Source: CAD feature listing. Evaluate the final solid. Frame: model axes, mm. A direction names the side the tool comes from. Give positions to 0.01 mm unless a question says otherwise; leave off trailing zeros. Loops run counter-clockwise (first coordinate to the right, second up) from the corner with the lowest first, then second, coordinate; pieces in that order, holes last. Notation, with made-up numbers: (-23.75, -25.75) -> (-6.75, -25.75) arc R8 cw to (-6.75, -15.75) -> close; hole circle Ø10 at (-24.5, 63.25). An arc over 180 degrees is marked (long way). Put each result on its own line as item: value.
```python
from build123d import *

# Parameters (mm, degrees)
SKETCH_1_W          = 48
SKETCH_1_H          = 69
EXTRUDE_1_DEPTH     = 2
SKETCH_2_W          = 60
SKETCH_2_H          = 81
EXTRUDE_2_DEPTH     = 2
SKETCH_3_W          = 48
SKETCH_3_H          = 69
CUT_EXTRUDE_1_DEPTH = 2
SKETCH_4_W          = 6
SKETCH_4_H          = 6
EXTRUDE_3_DEPTH     = 2
SKETCH_5_R          = 1.275
CUT_EXTRUDE_2_DEPTH = 2
FILLET_1_R          = 2


with BuildPart() as part:
    # 草图1 → 凸台-拉伸1 (new body)
    with BuildSketch(Plane(origin=(0, 0, 0), x_dir=(1, 0, 0), z_dir=(0, 1, 0))):
        Rectangle(SKETCH_1_W, SKETCH_1_H)
    extrude(amount=EXTRUDE_1_DEPTH)

    # 草图2 → 凸台-拉伸2 (add)
    with BuildSketch(Plane(origin=(0, 2, 0), x_dir=(1, 0, 0), z_dir=(0, 1, 0))):
        Rectangle(SKETCH_2_W, SKETCH_2_H)
    extrude(amount=-EXTRUDE_2_DEPTH)

    # 草图3 → 切除-拉伸1 (cut)
    with BuildSketch(Plane(origin=(0, 2, 0), x_dir=(1, 0, 0), z_dir=(0, 1, 0))):
        Rectangle(SKETCH_3_W, SKETCH_3_H)
    extrude(amount=-CUT_EXTRUDE_1_DEPTH, mode=Mode.SUBTRACT)

    # 草图4 → 凸台-拉伸3 (add)
    with BuildSketch(Plane.XZ):
        with Locations((-21, 31.5)):
            Rectangle(SKETCH_4_W, SKETCH_4_H)
        with Locations((21, 31.5)):
            Rectangle(SKETCH_4_W, SKETCH_4_H)
        with Locations((-21, -31.5)):
            Rectangle(SKETCH_4_W, SKETCH_4_H)
        with Locations((21, -31.5)):
            Rectangle(SKETCH_4_W, SKETCH_4_H)
    extrude(amount=-EXTRUDE_3_DEPTH)

    # 草图5 → 切除-拉伸2 (cut)
    with BuildSketch(Plane.XZ):
        with Locations((-21, 31.5)):
            Circle(SKETCH_5_R)
        with Locations((-21, -31.5)):
            Circle(SKETCH_5_R)
        with Locations((21, -31.5)):
            Circle(SKETCH_5_R)
        with Locations((21, 31.5)):
            Circle(SKETCH_5_R)
    extrude(amount=-CUT_EXTRUDE_2_DEPTH, mode=Mode.SUBTRACT)

    # 圆角1
    fillet_1_edges = [part.edges().sort_by_distance(p)[0] for p in [
        (30, 1, -40.5),
        (-30, 1, -40.5),
        (-30, 1, 40.5),
        (30, 1, 40.5),
        (-24, 1, 28.5),
        (-18, 1, 34.5),
        (-18, 1, 28.5),
        (24, 1, 28.5),
        (18, 1, 28.5),
        (18, 1, 34.5),
        (-24, 1, -28.5),
        (-18, 1, -28.5),
        (-18, 1, -34.5),
        (24, 1, -28.5),
        (18, 1, -34.5),
        (18, 1, -28.5),
    ]]
    fillet(fillet_1_edges, radius=FILLET_1_R)


solid = part.part
```
(1) Section A-A on z = -31.5. Return loops of the section in (x, y) (3 decimals), then the cut area to 3 significant figures.
Calculated:
outline: (-30, 0) -> (-22.275, 0) -> (-22.275, 2) -> (-30, 2) -> close; (-19.725, 0) -> (-18, 0) -> (-18, 2) -> (-19.725, 2) -> close; (18, 0) -> (19.725, 0) -> (19.725, 2) -> (18, 2) -> close; (22.275, 0) -> (30, 0) -> (30, 2) -> (22.275, 2) -> close
area: 37.8 mm²
(2) Reachability of faces 1 (the flat face through (0, 1, -40.5)), 2 (the flat face through (18, 1, -32)) from +Z, -Z, +X, -X, +Y, -Y: full face, straight path, thin tool, end or side. Return the list, or none.
Calculated:
face 1: -Z, +X, -X, +Y, -Y
face 2: +Y, -Y
(3) First-contact query: P1, Ø2, axis at x = 21, z = -31.5, coming from the -Y side. Flat tip, straight axial feed; report the tip coordinate or a pass-through.
Calculated:
P1: passes through
(4) Section D-D on x = -14. Return loops of the section in (y, z).
Calculated:
outline: (0, -40.5) -> (2, -40.5) -> (2, -34.5) -> (0, -34.5) -> close; (0, 34.5) -> (2, 34.5) -> (2, 40.5) -> (0, 40.5) -> close
(5) Line query: probe 1 along Z at (x, y) = (-21, 1.45) (3 decimals); probe 2 along X at (y, z) = (0.55, -21); probe 3 along Z at (x, y) = (-2.5, 1.5). Output: solid intervals per line, ascending. Write a range as from..to.
Calculated:
probe 1: z = -40.5..-32.775, -30.225..-28.5, 28.5..30.225, 32.775..40.5
probe 2: x = -30..-24, 24..30
probe 3: z = -40.5..-34.5, 34.5..40.5
(6) Section C-C on z = 1. Return loops of the section in (x, y).
Calculated:
outline: (-30, 0) -> (-24, 0) -> (-24, 2) -> (-30, 2) -> close; (24, 0) -> (30, 0) -> (30, 2) -> (24, 2) -> close
(7) Draft query along X for faces 3 (the flat face through (-24, 1, 0)), 4 (the cylindrical face through (-17.43, 1.01, -33.9)), 5 (the flat face through (0, 1, 40.5)), 6 (the flat face through (-30, 1, 1)). Return one class per face: released by +X, released by -X, zero draft, split by the parting line, or undercut.
Calculated:
face 3: undercut
face 4: undercut
face 5: zero draft
face 6: released by -X
(8) Section B-B on x = 21. Return loops of the section in (y, z) (3 decimals), then the cut area to 3 significant figures.
Calculated:
outline: (0, -40.5) -> (2, -40.5) -> (2, -32.775) -> (0, -32.775) -> close; (0, -30.225) -> (2, -30.225) -> (2, -28.5) -> (0, -28.5) -> close; (0, 28.5) -> (2, 28.5) -> (2, 30.225) -> (0, 30.225) -> close; (0, 32.775) -> (2, 32.775) -> (2, 40.5) -> (0, 40.5) -> close
area: 37.8 mm²
